Build history of the part. All positions in model axes, mm. Face numbers are marked on the shaded views. A direction names the side the tool comes from. Give positions to 0.01 mm unless a question says otherwise; leave off trailing zeros. Loops run counter-clockwise (first coordinate to the right, second up) from the corner with the lowest first, then second, coordinate; pieces in that order, holes last. Notation, with made-up numbers: M -8,23.5 L 25,23.5 A17 cw 25,43.5 Z; hole C 62,39.5 d7. An arc over 180 degrees is marked long. Answer as a JSON object with one key per item and string values. Group by question number.
1. Drop flat-ended pins along their axis: pin 1 Ø3.5 at (x, y) = (0, 0) entering from -Z; pin 2 Ø1.5 at (x, z) = (8, 1) entering from -Y; pin 3 Ø2 at (x, y) = (16.5, 3) entering from -Z; pin 4 Ø0.7 at (y, z) = (-6.5, 2.5) entering from -X. Give the stop position or say it passes through.
2. Slice it at B-B (x = 1.5). List the corners of the cut face in (y, z) (3 decimals).
3. Slice it at D-D (x = 4.25). List the corners of the cut face in (y, z) (3 decimals).
4. Slice it at A-A (y = 0.75). List the corners of the cut face in (x, z) (3 decimals), then the cut area to 3 significant figures.
5. 3-axis set-ups, long thin cutter, end or side, ignore diameter. For the marked faces 1 and 2: which of +Z, -Z, +X, -X, +Y, -Y reach the whole face in a straight line?
6. Mould opens along X. For the marked faces 3, 4, 5 and 6 say: released by +X, released by -X, zero draft, split by the parting line, or undercut.
7. Slice it at C-C (z = 2.5). Give the number of separate pieces and of enclosed holes in the cut face, then the cut area to 3 significant figures.
8. Drill centre lines: line 1 along Y through (x, z) = (0, 2.55); line 2 along X through (y, z) = (9, 0.8); line 3 along X through (y, z) = (8.75, 0.55). Where is each one in solid material? Low to high. Write a range as [from, to].
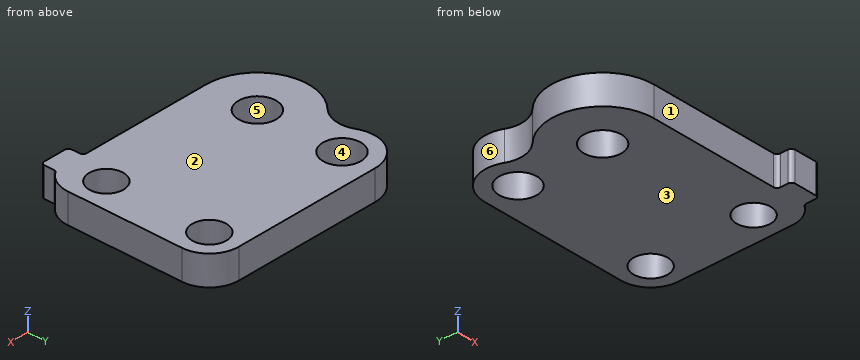
from build123d import *

# Parameters (mm, degrees)
SKETCH3_R           = 1.8415
SKETCH3_R_2         = 2.0399375
BOSS_EXTRUDE1_DEPTH = 3.175
FILLET1_R           = 3.175
FILLET2_R           = 0.396875


with BuildPart() as part:
    # Sketch3 → Boss-Extrude1 (new body)
    with BuildSketch(Plane.XY):
        with BuildLine():
            Line((0, -5.55625), (14.2875, -5.55625))
            Line((14.2875, -5.55625), (14.2875, -7.18185))
            Line((14.2875, -7.18185), (17.4625, -7.18185))
            Line((17.4625, -7.18185), (17.4625, -5.55625))
            Line((17.4625, -5.55625), (19.05, -5.55625))
            Line((19.05, -5.55625), (19.05, 12.7))
            Line((19.05, 12.7), (0, 12.7))
            ThreePointArc((0, 12.7), (-3.017240851, 11.039812386), (-3.229688204, 7.602541465))
            ThreePointArc((-3.229688204, 7.602541465), (-2.975666517, 5.684416089), (-3.882150485, 3.975024739))
            ThreePointArc((-3.882150485, 3.975024739), (-5.145782024, -2.095910644), (0, -5.55625))
        make_face()
        with Locations((15.875, 9.525)):
            Circle(SKETCH3_R, mode=Mode.SUBTRACT)
        with Locations((15.875, -1.5875)):
            Circle(SKETCH3_R, mode=Mode.SUBTRACT)
        with Locations((0, 9.128125)):
            Circle(SKETCH3_R_2, mode=Mode.SUBTRACT)
        Circle(SKETCH3_R_2, mode=Mode.SUBTRACT)
    extrude(amount=BOSS_EXTRUDE1_DEPTH)

    # Fillet1
    # the kernel refuses this fillet: 3.175 mm, written as the material it takes off along each edge
    with BuildSketch(Plane(origin=(19.05, -5.55625, -6.874076643), x_dir=(-1, 0, 0), z_dir=(0, 0, 1))) as fillet1_piece_1:
        with BuildLine():
            CenterArc((3.175, -2.749630657), FILLET1_R, 120, 60)
            Line((0, -2.749630657), (-0.0635, -2.749630657))
            Line((-0.0635, -2.749630657), (-0.0635, 0))
            Line((-0.0635, 0), (0, 0.0635))
            ThreePointArc((0, 0.0635), (0.79375, 0.0635), (1.55575, 0.054992613))
            Line((1.55575, 0.054992613), (1.5875, 0))
        make_face()
    extrude(amount=16.923153285, mode=Mode.SUBTRACT)
    with BuildSketch(Plane(origin=(19.05, 12.7, -7.9375), x_dir=(0, -1, 0), z_dir=(0, 0, 1))) as fillet1_piece_2:
        with BuildLine():
            CenterArc((FILLET1_R, -FILLET1_R), FILLET1_R, 90, 90)
            Line((0, -FILLET1_R), (-FILLET1_R * 0.02, -FILLET1_R))
            Line((-FILLET1_R * 0.02, -FILLET1_R), (-FILLET1_R * 0.02, FILLET1_R * 0.02))
            Line((-FILLET1_R * 0.02, FILLET1_R * 0.02), (FILLET1_R, FILLET1_R * 0.02))
            Line((FILLET1_R, FILLET1_R * 0.02), (FILLET1_R, 0))
        make_face()
    extrude(amount=19.05, mode=Mode.SUBTRACT)

    # Fillet2
    fillet2_edges = [part.edges().sort_by_distance(p)[0] for p in [
        (17.4625, -5.55625, 1.5875),
        (17.4625, -7.18185, 1.5875),
        (14.2875, -7.18185, 1.5875),
        (14.2875, -5.55625, 1.5875),
    ]]
    fillet(fillet2_edges, radius=FILLET2_R)


solid = part.part
Established:
{
 "1": {"pin 1": "passes through", "pin 2": "stops at y = -5.56", "pin 3": "stops at z = 0", "pin 4": "stops at x = 14.29"},
 "2": {"outline": "M -5.556,0 L -1.383,0 L -1.383,3.175 L -5.556,3.175 Z; M 1.383,0 L 7.746,0 L 7.746,3.175 L 1.383,3.175 Z; M 10.511,0 L 12.7,0 L 12.7,3.175 L 10.511,3.175 Z"},
 "3": {"outline": "M -5.556,0 L 12.7,0 L 12.7,3.175 L -5.556,3.175 Z"},
 "4": {"outline": "M -5.505,0 L -1.897,0 L -1.897,3.175 L -5.505,3.175 Z; M 1.897,0 L 19.05,0 L 19.05,3.175 L 1.897,3.175 Z", "area": "65.9 mm^2"},
 "5": {"face 1": "+Z, -Z, -X, -Y", "face 2": "+Z, +X, -X, +Y, -Y"},
 "6": {"face 3": "zero draft", "face 4": "undercut", "face 5": "undercut", "face 6": "released by -X"},
 "7": {"separate pieces": "1", "enclosed holes": "4", "area": "373 mm^2"},
 "8": {"line 1": "y = [-5.56, -2.04], [2.04, 7.09], [11.17, 12.7]", "line 2": "x = [-3.57, -2.04], [2.04, 14.11], [17.64, 19.05]", "line 3": "x = [-3.55, -2], [2, 14.2], [17.55, 19.05]"}
}
